```python
from build123d import *

# Parameters (mm, degrees)
CROQUIS1_W              = 500
CROQUIS1_H              = 920
SALIENTE_EXTRUIR1_DEPTH = 15
CROQUIS2_R              = 2.5
CORTAR_EXTRUIR1_DEPTH   = 524.760441423
CROQUIS3_R              = 2.5
CORTAR_EXTRUIR2_DEPTH   = 680.577074363
CROQUIS5_R              = 1.75
CROQUIS5_W              = 30
CROQUIS5_H              = 36
CORTAR_EXTRUIR3_DEPTH   = 524.760441423
CROQUIS6_W              = 68.576294335
CROQUIS6_H              = 90.214445459
SALIENTE_EXTRUIR2_DEPTH = 15
CROQUIS7_W              = 40
CROQUIS7_H              = 40
CORTAR_EXTRUIR4_DEPTH   = 15
CORTAR_EXTRUIR5_START   = -15
CROQUIS8_W              = 20.35
CROQUIS8_H              = 920
CROQUIS8_W_2            = 24.91
CORTAR_EXTRUIR5_DEPTH   = 15


with BuildPart() as part:
    # Croquis1 → Saliente-Extruir1 (new body)
    with BuildSketch(Plane.XY):
        Rectangle(CROQUIS1_W, CROQUIS1_H)
    extrude(amount=SALIENTE_EXTRUIR1_DEPTH)

    # Croquis2 → Cortar-Extruir1 (cut, through all)
    with BuildSketch(Plane.XY.offset(15)):
        with Locations((0, -265)):
            Circle(CROQUIS2_R)
        with Locations((0, 395)):
            Circle(CROQUIS2_R)
    extrude(amount=-CORTAR_EXTRUIR1_DEPTH, mode=Mode.SUBTRACT)

    # Croquis3 → Cortar-Extruir2 (cut, through all)
    with BuildSketch(Plane(origin=(250, 0, 0), x_dir=(0, 0, -1), z_dir=(1, 0, 0))):
        with Locations((-7.5, 445)):
            Circle(CROQUIS3_R)
        with Locations(Location((-7.5, -445, 0), (0, 0, 180))):
            Circle(CROQUIS3_R)
    extrude(amount=-CORTAR_EXTRUIR2_DEPTH, mode=Mode.SUBTRACT)

    # Croquis5 → Cortar-Extruir3 (cut, through all)
    with BuildSketch(Plane(origin=(0, 0, 0), x_dir=(-1, 0, 0), z_dir=(0, 0, -1))):
        with Locations((-74.2, 208.5)):
            Circle(CROQUIS5_R)
        with Locations((-74.2, 278.5)):
            Circle(CROQUIS5_R)
        with Locations(Location((-125.8, 278.5, 0), (0, 0, 180))):
            Circle(CROQUIS5_R)
        with Locations(Location((-125.8, 208.5, 0), (0, 0, 180))):
            Circle(CROQUIS5_R)
        with Locations((125.8, 208.5)):
            Circle(CROQUIS5_R)
        with Locations((125.8, 278.5)):
            Circle(CROQUIS5_R)
        with Locations(Location((74.2, 278.5, 0), (0, 0, 180))):
            Circle(CROQUIS5_R)
        with Locations(Location((74.2, 208.5, 0), (0, 0, 180))):
            Circle(CROQUIS5_R)
        with Locations((125.8, -31.5)):
            Circle(CROQUIS5_R)
        with Locations((125.8, 38.5)):
            Circle(CROQUIS5_R)
        with Locations(Location((74.2, 38.5, 0), (0, 0, 180))):
            Circle(CROQUIS5_R)
        with Locations(Location((74.2, -31.5, 0), (0, 0, 180))):
            Circle(CROQUIS5_R)
        with Locations((125.8, -251.5)):
            Circle(CROQUIS5_R)
        with Locations((125.8, -181.5)):
            Circle(CROQUIS5_R)
        with Locations(Location((74.2, -181.5, 0), (0, 0, 180))):
            Circle(CROQUIS5_R)
        with Locations(Location((74.2, -251.5, 0), (0, 0, 180))):
            Circle(CROQUIS5_R)
        with Locations((-74.2, -31.5)):
            Circle(CROQUIS5_R)
        with Locations((-74.2, 38.5)):
            Circle(CROQUIS5_R)
        with Locations(Location((-125.8, 38.5, 0), (0, 0, 180))):
            Circle(CROQUIS5_R)
        with Locations(Location((-125.8, -31.5, 0), (0, 0, 180))):
            Circle(CROQUIS5_R)
        with Locations((-74.2, -251.5)):
            Circle(CROQUIS5_R)
        with Locations((-74.2, -181.5)):
            Circle(CROQUIS5_R)
        with Locations(Location((-125.8, -181.5, 0), (0, 0, 180))):
            Circle(CROQUIS5_R)
        with Locations(Location((-125.8, -251.5, 0), (0, 0, 180))):
            Circle(CROQUIS5_R)
        with Locations((100, 220)):
            Rectangle(CROQUIS5_W, CROQUIS5_H)
        with Locations((-100, 220)):
            Rectangle(CROQUIS5_W, CROQUIS5_H)
        with Locations((100, -20)):
            Rectangle(CROQUIS5_W, CROQUIS5_H)
        with Locations((100, -240)):
            Rectangle(CROQUIS5_W, CROQUIS5_H)
        with Locations((-100, -20)):
            Rectangle(CROQUIS5_W, CROQUIS5_H)
        with Locations((-100, -240)):
            Rectangle(CROQUIS5_W, CROQUIS5_H)
    extrude(amount=-CORTAR_EXTRUIR3_DEPTH, mode=Mode.SUBTRACT)

    # Croquis6 → Saliente-Extruir2 (add)
    with BuildSketch(Plane(origin=(0, 0, 0), x_dir=(-1, 0, 0), z_dir=(0, 0, -1))):
        with Locations((-98.305946691, 244.444644428)):
            Rectangle(CROQUIS6_W, CROQUIS6_H)
    extrude(amount=-SALIENTE_EXTRUIR2_DEPTH)

    # Croquis7 → Cortar-Extruir4 (cut)
    with BuildSketch(Plane(origin=(0, 0, 0), x_dir=(-1, 0, 0), z_dir=(0, 0, -1))):
        with Locations((-64, 222)):
            Rectangle(CROQUIS7_W, CROQUIS7_H)
        with Locations((-136, 222)):
            Rectangle(CROQUIS7_W, CROQUIS7_H)
    extrude(amount=-CORTAR_EXTRUIR4_DEPTH, mode=Mode.SUBTRACT)

    # Croquis8 → Cortar-Extruir5 (cut)
    with BuildSketch(Plane(origin=(0, 0, 0), x_dir=(-1, 0, 0), z_dir=(0, 0, -1)).offset(CORTAR_EXTRUIR5_START)):
        with Locations((239.825, 0)):
            Rectangle(CROQUIS8_W, CROQUIS8_H)
        with Locations((-237.545, 0)):
            Rectangle(CROQUIS8_W_2, CROQUIS8_H)
    extrude(amount=CORTAR_EXTRUIR5_DEPTH, mode=Mode.SUBTRACT)


solid = part.part
```
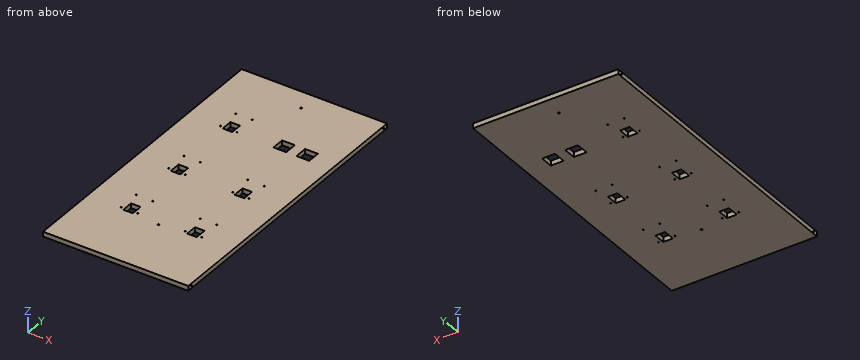
The model under review builds one solid part; all positions refer to its coordinate system, in mm. Give positions to 0.01 mm unless a question says otherwise; leave off trailing zeros. Write each loop counter-clockwise with the first axis right and the second up, starting at its lowest first coordinate (ties: lowest second). Pieces come first, ordered by that corner, then holes. Notation, with made-up numbers: M -20,65.5 L -7,65.5 A25 ccw -7,101.5 Z; hole C -4,81.5 d1. An arc over 180 degrees is marked long. Write item = value, one per line. Start each with the question number.
Q1. For line 1 (X direction, y = -29, z = 1.25); line 2 (Y direction, x = -108, z = 4.25); line 3 (Y direction, x = 73.5, z = 2.5), list the stretches that pass through material, from the lowest coordinate up.
Q2. We need section B-B (z = 7.5). Give the number of separate pieces and of enclosed holes in the cut face, plus the area to 3 significant figures.
Q3. Clearance check with flat-ended pins moving along their axes: pin 1 (3 mm diameter, centred on x = -74.2, y = -251.5, fed in from -Z); pin 2 (4.5 mm diameter, centred on x = -125.8, y = -251.5, fed in from +Z). State where each tip first meets the part, or that it passes through.
Q4. We need section A-A (x = 61.5). State the section outline as (y, z) points.
Result set:
q1.line_1 = -229.65 to -115, -85 to 85, 115 to 225.09
q1.line_2 = -460 to -258, -222 to -38, -2 to 202, 238 to 460
q1.line_3 = -460 to -253.1, -249.9 to -183.1, -179.9 to -33.1, -29.9 to 36.9, 40.1 to 202, 242 to 460
q2.separate_pieces = 3
q2.enclosed_holes = 29
q2.area = 405,000 mm2
q3.pin_1 = through
q3.pin_2 = 15
q4.outline = M -460,0 L 202,0 L 202,15 L -460,15 Z; M 242,0 L 460,0 L 460,15 L 242,15 Z; hole C -445,7.5 d5; hole C 445,7.5 d5
